from build123d import *

# Parameters (mm, degrees)
SKETCH_1_W                   = 30
SKETCH_1_H                   = 30
EXTRUDE_1_DEPTH              = 5
SKETCH_2_W                   = 3
SKETCH_2_H                   = 3
EXTRUDE_2_DEPTH              = 10
EXTRUDE_3_DEPTH              = 7
CUT_EXTRUDE_1_DEPTH          = 10
CUT_EXTRUDE_2_DEPTH          = 10
HOLE_WIZARD_M4_1_D           = 4.5
HOLE_WIZARD_M4_1_CBORE_D     = 8
HOLE_WIZARD_M4_1_CBORE_DEPTH = 4
EXTRUDE_4_DEPTH              = 10
CHAMFER_1_SIZE               = 1
CUT_EXTRUDE_4_DEPTH          = 10
EXTRUDE_5_DEPTH              = 4
EXTRUDE_6_DEPTH              = 4


with BuildPart() as part:
    # 스케치1 → 보스-돌출1 (new body)
    with BuildSketch(Plane.XY):
        Rectangle(SKETCH_1_W, SKETCH_1_H)
    extrude(amount=EXTRUDE_1_DEPTH)

    # 스케치2 → 보스-돌출2 (add)
    with BuildSketch(Plane.XY.offset(5)):
        with Locations((-13.5, 13.5)):
            Rectangle(SKETCH_2_W, SKETCH_2_H)
    extrude(amount=EXTRUDE_2_DEPTH)

    # 스케치2<3> → 보스-돌출3 (add)
    with BuildSketch(Plane.XY.offset(5)):
        Polygon((15, 15), (11, 15), (11, -11), (-15, -11), (-15, -15), (15, -15), align=None)
    extrude(amount=EXTRUDE_3_DEPTH)

    # 스케치3 → 컷-돌출1 (cut)
    with BuildSketch(Plane(origin=(-12, 0, 0), x_dir=(0, 0, -1), z_dir=(1, 0, 0))):
        Polygon((-15, 13.5), (-5, 12), (-15, 12), align=None)
    extrude(amount=-CUT_EXTRUDE_1_DEPTH, mode=Mode.SUBTRACT)

    # 스케치4 → 컷-돌출2 (cut)
    with BuildSketch(Plane(origin=(0, 15, 0), x_dir=(1, 0, 0), z_dir=(0, 1, 0))):
        Polygon((-12, -15), (-12, -5), (-13.5, -15), align=None)
    extrude(amount=-CUT_EXTRUDE_2_DEPTH, mode=Mode.SUBTRACT)

    # M4 소켓 머리 캡 나사용 카운터보어1 (through all)
    with Locations(Plane.XY.offset(5)):
        with Locations((0, 0)):
            CounterBoreHole(HOLE_WIZARD_M4_1_D / 2, HOLE_WIZARD_M4_1_CBORE_D / 2, HOLE_WIZARD_M4_1_CBORE_DEPTH)

    # 스케치8 → 보스-돌출4 (add)
    with BuildSketch(Plane(origin=(0, 0, 0), x_dir=(-1, 0, 0), z_dir=(0, 0, -1))):
        with BuildLine():
            Line((-3.05, 15), (3.05, 15))
            Line((3.05, 15), (3.05, 12.5))
            Line((3.05, 12.5), (5.05, 12.5))
            Line((5.05, 12.5), (5.05, 6.454957169))
            ThreePointArc((5.05, 6.454957169), (0, 4.5), (-5.05, 6.454957169))
            Line((-5.05, 6.454957169), (-5.05, 12.5))
            Line((-5.05, 12.5), (-3.05, 12.5))
            Line((-3.05, 12.5), (-3.05, 15))
        make_face()
        with BuildLine():
            Line((15, 3.05), (15, -3.05))
            Line((15, -3.05), (12.5, -3.05))
            Line((12.5, -3.05), (12.5, -5.05))
            Line((12.5, -5.05), (6.454957169, -5.05))
            ThreePointArc((6.454957169, -5.05), (4.5, 0), (6.454957169, 5.05))
            Line((6.454957169, 5.05), (12.5, 5.05))
            Line((12.5, 5.05), (12.5, 3.05))
            Line((12.5, 3.05), (15, 3.05))
        make_face()
        with BuildLine():
            Line((3.05, -15), (-3.05, -15))
            Line((-3.05, -15), (-3.05, -12.5))
            Line((-3.05, -12.5), (-5.05, -12.5))
            Line((-5.05, -12.5), (-5.05, -6.454957169))
            ThreePointArc((-5.05, -6.454957169), (0, -4.5), (5.05, -6.454957169))
            Line((5.05, -6.454957169), (5.05, -12.5))
            Line((5.05, -12.5), (3.05, -12.5))
            Line((3.05, -12.5), (3.05, -15))
        make_face()
        with BuildLine():
            Line((-15, -3.05), (-15, 3.05))
            Line((-15, 3.05), (-12.5, 3.05))
            Line((-12.5, 3.05), (-12.5, 5.05))
            Line((-12.5, 5.05), (-6.454957169, 5.05))
            ThreePointArc((-6.454957169, 5.05), (-4.5, 0), (-6.454957169, -5.05))
            Line((-6.454957169, -5.05), (-12.5, -5.05))
            Line((-12.5, -5.05), (-12.5, -3.05))
            Line((-12.5, -3.05), (-15, -3.05))
        make_face()
    extrude(amount=EXTRUDE_4_DEPTH)

    # 모따기1
    chamfer_1_edges = [part.edges().sort_by_distance(p)[0] for p in [
        (-13.75, -3.05, -10),
        (-15, 0, -10),
        (-13.75, 3.05, -10),
        (-12.5, 4.05, -10),
        (-9.477478584, 5.05, -10),
        (-4.5, 0, -10),
        (-9.477478584, -5.05, -10),
        (-12.5, -4.05, -10),
        (3.05, -13.75, -10),
        (0, -15, -10),
        (-3.05, -13.75, -10),
        (-4.05, -12.5, -10),
        (-5.05, -9.477478584, -10),
        (0, -4.5, -10),
        (5.05, -9.477478584, -10),
        (4.05, -12.5, -10),
        (13.75, 3.05, -10),
        (15, 0, -10),
        (13.75, -3.05, -10),
        (12.5, -4.05, -10),
        (9.477478584, -5.05, -10),
        (4.5, 0, -10),
        (9.477478584, 5.05, -10),
        (12.5, 4.05, -10),
        (-3.05, 13.75, -10),
        (0, 15, -10),
        (3.05, 13.75, -10),
        (4.05, 12.5, -10),
        (5.05, 9.477478584, -10),
        (0, 4.5, -10),
        (-5.05, 9.477478584, -10),
        (-4.05, 12.5, -10),
    ]]
    chamfer(chamfer_1_edges, length=CHAMFER_1_SIZE)

    # 스케치9 → 컷-돌출4 (cut)
    with BuildSketch(Plane(origin=(0, 0, -10), x_dir=(-1, 0, 0), z_dir=(0, 0, -1))):
        Polygon((-6.459146565, 15), (-6.459146565, 5.734562816), (1.656191427, 2.380775176), (5.83807478, -6.065801101), (15, -6.065801101), (15, 15), align=None)
    extrude(amount=-CUT_EXTRUDE_4_DEPTH, mode=Mode.SUBTRACT)

    # 스케치11 → 보스-돌출5 (add)
    with BuildSketch(Plane.XZ.offset(15)):
        Polygon((-15, 12), (-9, 20), (15, 20), (15, 12), align=None)
    extrude(amount=-EXTRUDE_5_DEPTH)

    # 스케치12 → 보스-돌출6 (add)
    with BuildSketch(Plane(origin=(15, 0, 0), x_dir=(0, 0, -1), z_dir=(1, 0, 0))):
        Polygon((-12, -11), (-12, 15), (-20, 9), (-20, -11), align=None)
    extrude(amount=-EXTRUDE_6_DEPTH)


solid = part.part
For this review, take the finished solid that the model builds, in its own axes (mm). A direction names the side the tool comes from. Round coordinates to 2 decimals unless told otherwise and drop trailing zeros. Write each loop counter-clockwise with the first axis right and the second up, starting at its lowest first coordinate (ties: lowest second). Pieces come first, ordered by that corner, then holes. Notation, with made-up numbers: M -22.5,57.25 L -12.5,57.25 A22 cw -12.5,78.25 Z; hole C 36.5,4.5 d11. An arc over 180 degrees is marked long. Write item = value, one per line. Start each with the question number.
(1) For faces 4 (the face through (-5.05, -9, -4)), 5 (the face through (9.44, -4.54, -9.51)), 6 (the face through (-12, -13, 16)), list the 3-axis set-ups (+Z, -Z, +X, -X, +Y, -Y) from which the entire face can be reached by the end or side of a thin tool; tool diameter is ignored.
(2) We need section A-A (x = 0). Give the boundary of the cut face in (y, z), then the cut area to 4 significant figures.
(3) Clearance check with flat-ended pins moving along their axes: pin 1 Ø5 at (y, z) = (-9.5, -4.5) entering from +X; pin 2 Ø3 at (x, z) = (9, -6.5) entering from +Y; pin 3 Ø3 at (x, y) = (5, 8) entering from +Z; pin 4 Ø4 at (x, y) = (0, 0) entering from +Z. State where each tip first meets the part, or that it passes through.
(4) We need section D-D (x = 8). Give the boundary of the cut face in (y, z), then the cut area to 3 significant figures.
(5) The part is to be moulded in two halves that separate along Y. For faces 1 (the face through (-13.81, 12.76, 10.07)), 2 (the face through (13, 12, 16)), 3 (the face through (15, 0, 9)), say which applies: +Y half, -Y half, draft (parallel to the pull), parting line (faces both ways), or undercut.
(6) We need section C-C (y = 0). Give the boundary of the cut face in (x, z), then the cut area to 4 significant figures.
(7) For line 1 along Y through (x, z) = (0, 0.7); line 2 along Y through (x, z) = (0, 2.35); line 3 along Z through (x, y) = (-4.75, 10.25), list the stretches that pass through material, from the lowest coordinate up.
(8) We need section B-B (z = -4). Give the boundary of the cut face in (x, y).
Results found:
q1.face_4 = -Z, -X, +Y, -Y
q1.face_5 = -Z, +X, -Y
q1.face_6 = +Z, -X, -Y
q2.outline = M -15,-9 L -14,-10 L -5.5,-10 L -4.5,-9 L -4.5,0 L -2.25,0 L -2.25,1 L -4,1 L -4,5 L -11,5 L -11,20 L -15,20 Z; M 2.25,0 L 15,0 L 15,5 L 4,5 L 4,1 L 2.25,1 Z
q2.area = 277.5 mm²
q3.pin_1 = 5.05
q3.pin_2 = 5.05
q3.pin_3 = 5
q3.pin_4 = through
q4.outline = M -15,0 L -5.05,0 L -5.05,-9 L -4.05,-10 L 4.05,-10 L 5.05,-9 L 5.05,0 L 15,0 L 15,5 L -11,5 L -11,20 L -15,20 Z
q4.area = 310 mm²
q5.face_1 = undercut
q5.face_2 = +Y half
q5.face_3 = draft
q6.outline = M -15,0 L -2.25,0 L -2.25,1 L -4,1 L -4,5 L -15,5 Z; M 2.25,0 L 4.5,0 L 4.5,-9 L 5.5,-10 L 14,-10 L 15,-9 L 15,20 L 11,20 L 11,5 L 4,5 L 4,1 L 2.25,1 Z
q6.area = 277.5 mm²
q7.line_1 = -15 to -2.25, 2.25 to 15
q7.line_2 = -15 to -4, 4 to 15
q7.line_3 = 0 to 5
q8.outline = M -5.05,-12.5 L -3.05,-12.5 L -3.05,-15 L 3.05,-15 L 3.05,-12.5 L 5.05,-12.5 L 5.05,-6.45 A7.5 ccw -5.05,-6.45 Z; M 6.45,-5.05 L 12.5,-5.05 L 12.5,-3.05 L 15,-3.05 L 15,3.05 L 12.5,3.05 L 12.5,5.05 L 6.45,5.05 A7.5 ccw Z
